Drawing for the job (mm, zero at the part's lowest x, y, z). Give positions to 0.01 mm unless a question says otherwise; leave off trailing zeros. Write each loop counter-clockwise with the first axis right and the second up, starting at its lowest first coordinate (ties: lowest second). Pieces come first, ordered by that corner, then holes. Notation, with made-up numbers: M 34.5,-20 L 76.5,-20 A13 ccw 76.5,-13 Z; hole C 8,26.5 d8. An arc over 180 degrees is marked long. Answer as a JSON object with one key per item and string values. Group by question number.
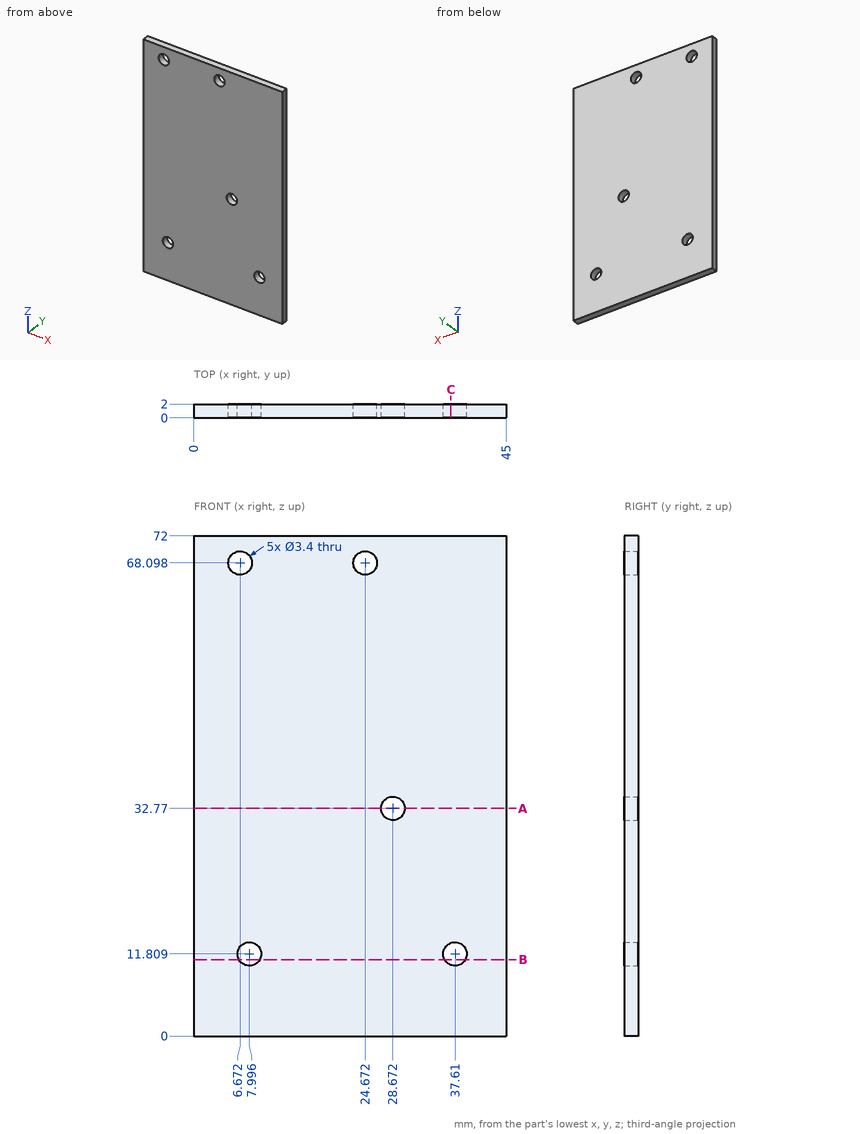
Q1. Drop a flat-ended pin along its axis: P1, Ø5.5, axis at x = 37.61, z = 11.81, coming from the +Y side. Give the stop position or say it passes through.
Q2. Slice it at A-A, the plane z = 32.77. Write the cut outline in (x, y).
Q3. Wall check: L1, parallel to X at y = 1.25, z = 32.77; L2, parallel to X at y = 0.45, z = 11.5 (1 decimal); L3, parallel to Z at x = 25.5, y = 0.35. Give the ranges that are in metal, low to high.
Q4. Slice it at B-B, the plane z = 11. Write the cut outline in (x, y) (1 decimal).
Q5. Slice it at C-C, the plane x = 37. Write the cut outline in (y, z), then the cut area to 3 significant figures.
Solved:
{
 "1": {"P1": "stops at y = 2"},
 "2": {"outline": "M 0,0 L 26.97,0 L 26.97,2 L 0,2 Z; M 30.37,0 L 45,0 L 45,2 L 30.37,2 Z"},
 "3": {"L1": "x = 0 to 26.97, 30.37 to 45", "L2": "x = 0 to 6.3, 9.7 to 35.9, 39.3 to 45", "L3": "z = 0 to 66.61, 69.58 to 72"},
 "4": {"outline": "M 0,0 L 6.5,0 L 6.5,2 L 0,2 Z; M 9.5,0 L 36.1,0 L 36.1,2 L 9.5,2 Z; M 39.1,0 L 45,0 L 45,2 L 39.1,2 Z"},
 "5": {"outline": "M 0,0 L 2,0 L 2,10.22 L 0,10.22 Z; M 0,13.4 L 2,13.4 L 2,72 L 0,72 Z", "area": "138 mm²"}
}
